```python
from build123d import *

# Parameters (mm, degrees)
SKETCH1_R           = 30
BOSS_EXTRUDE1_DEPTH = 3
SKETCH2_R           = 30
SKETCH2_R_2         = 27
BOSS_EXTRUDE2_DEPTH = 250
CUT_EXTRUDE1_DEPTH  = 44


with BuildPart() as part:
    # Sketch1 → Boss-Extrude1 (new body)
    with BuildSketch(Plane(origin=(0, 0, 0), x_dir=(1, 0, 0), z_dir=(0, 1, 0))):
        Circle(SKETCH1_R)
    extrude(amount=BOSS_EXTRUDE1_DEPTH)

    # Sketch2 → Boss-Extrude2 (add)
    with BuildSketch(Plane(origin=(0, 3, 0), x_dir=(1, 0, 0), z_dir=(0, 1, 0))):
        Circle(SKETCH2_R)
        Circle(SKETCH2_R_2, mode=Mode.SUBTRACT)
    extrude(amount=BOSS_EXTRUDE2_DEPTH)

    # Sketch3 → Cut-Extrude1 (cut)
    with BuildSketch(Plane.XZ):
        Polygon((-1.5, 0), (-1.5, 12.25), (1.5, 12.25), (1.5, 0), (1.5, -12.25), (-1.5, -12.25), align=None)
    extrude(amount=-CUT_EXTRUDE1_DEPTH, mode=Mode.SUBTRACT)


solid = part.part
```
Build history of the part. All positions in model axes, mm. A direction names the side the tool comes from. Coordinates: 2 decimals unless noted, no trailing zeros. Order: outer loops, then holes, each group sorted by start corner. A loop starts at its lowest first (then second) coordinate and runs counter-clockwise, first axis right, second up. Notation, with made-up numbers: M 76,-12.5 L 108,-12.5 A31 cw 108,20.5 Z; hole C -30,83 d4. An arc over 180 degrees is marked long. One line per question, with ' | ' between items. Start each with the question number.
1. Mould opens along Z. For faces 1 (the face through (-29.97, 124.73, -1.32)), 2 (the face through (-25, 253, -11)), 3 (the face through (-5.85, 126.25, 26.36)) say: +Z half, -Z half, draft (parallel to the pull), parting line (faces both ways), or undercut.
2. Wall check: line 1 along Z through (x, y) = (0, 78); line 2 along Y through (x, z) = (9, 25). Give the ranges that are in metal, low to high. Write a range as [from, to].
3. Cut at A-A (z = 0). Write the cut outline in (x, y).
4. Cut at C-C (x = -7). Write the cut outline in (y, z), plus the area to 3 significant figures.
5. Tool access for faces 4 (the face through (6, 0, 0)), 5 (the face through (6, 3, 0)): list every direction of +Z, -Z, +X, -X, +Y, -Y with a clear straight run to the whole face (end or side of a thin tool).
6. Flat gauge pins, fed straight in: P1, Ø5, axis at x = -5, y = 91, coming from the +Z side; P2, Ø5, axis at y = 88, z = -6, coming from the +X side; P3, Ø1.5, axis at x = 12, y = 96.5, coming from the +Z side. Where does each tip first touch, or does it go through?
7. Cut at D-D (z = -17). Write the cut outline in (x, y).
8. Cut at B-B (y = 57.5). Write the cut outline in (x, z).
The answers:
1) face 1: parting line | face 2: draft | face 3: undercut
2) line 1: z = [-30, -27], [27, 30] | line 2: y = [0, 3]
3) outline: M -30,0 L -1.5,0 L -1.5,3 L -27,3 L -27,253 L -30,253 Z; M 1.5,0 L 30,0 L 30,253 L 27,253 L 27,3 L 1.5,3 Z
4) outline: M 0,-29.17 L 253,-29.17 L 253,-26.08 L 3,-26.08 L 3,26.08 L 253,26.08 L 253,29.17 L 0,29.17 Z | area: 1,720 mm2
5) face 4: +Z, -Z, +X, -X, -Y | face 5: +Y
6) P1: stops at z = 29.9 | P2: stops at x = 29.8 | P3: stops at z = 27.81
7) outline: M -24.72,0 L 24.72,0 L 24.72,253 L 20.98,253 L 20.98,3 L -20.98,3 L -20.98,253 L -24.72,253 Z
8) outline: C 0,0 d60; hole C 0,0 d54
